from build123d import *

# Parameters (mm, degrees)
SKETCH_1_R             = 1.6
EXTRUDE_2_DEPTH        = 3
SKETCH_2_W             = 5
SKETCH_2_H             = 5.5
CUT_EXTRUDE_1_DEPTH    = 5
PATTERN_LINEAR_1_COUNT = 2
PATTERN_LINEAR_1_PITCH = 62.5


with BuildPart() as part:
    # 草图1 → 凸台-拉伸2 (new body)
    with BuildSketch(Plane.XY):
        Polygon((137.75, -25.25), (38.57, -25.25), (-17.446603057, -105.25), (137.75, -105.25), align=None)
        with Locations((36.773595123, -45.25)):
            Circle(SKETCH_1_R, mode=Mode.SUBTRACT)
        with Locations((1.763218213, -95.25)):
            Circle(SKETCH_1_R, mode=Mode.SUBTRACT)
        with Locations((127.75, -35.25)):
            Circle(SKETCH_1_R, mode=Mode.SUBTRACT)
        with Locations((127.75, -95.25)):
            Circle(SKETCH_1_R, mode=Mode.SUBTRACT)
    extrude(amount=EXTRUDE_2_DEPTH)

    # 草图2 → 切除-拉伸1 (cut)
    with BuildSketch(Plane.XY.offset(3)):
        with Locations((98.25, -97.500011017)):
            Rectangle(SKETCH_2_W, SKETCH_2_H)
        with Locations((48.25, -97.500011017)):
            Rectangle(SKETCH_2_W, SKETCH_2_H)
    cut_extrude_1 = extrude(amount=-CUT_EXTRUDE_1_DEPTH, mode=Mode.SUBTRACT)

    # 阵列(线性)1: 切除-拉伸1 ×2
    with Locations(*[(0, i * PATTERN_LINEAR_1_PITCH, 0) for i in range(1, PATTERN_LINEAR_1_COUNT)]):
        add(cut_extrude_1, mode=Mode.SUBTRACT)


solid = part.part
Input: part model. Units: mm. Frame: model coordinates. A direction names the side the tool comes from. Round coordinates to 2 decimals unless told otherwise and drop trailing zeros. Order: outer loops, then holes, each group sorted by start corner. A loop starts at its lowest first (then second) coordinate and runs counter-clockwise, first axis right, second up. Notation, with made-up numbers: (23, 7) - (31, 7) arc R19 ccw to (31, 16) - close; hole circle Ø8 at (-19.75, 36). An arc over 180 degrees is marked (long way). Answer as a JSON object with one key per item and string values. Group by question number.
(1) Cut plane C-C (y = -35.25). Return loops of the section in (x, z), then the cut area to 3 significant figures.
(2) Cut plane D-D (x = 48.5). Return loops of the section in (y, z), then the cut area to 3 significant figures.
(3) Reachability of faces 1 (the face through (100.75, -98, 2)), 2 (the face through (76, -65, 3)) from +Z, -Z, +X, -X, +Y, -Y: full face, straight path, thin tool, end or side. Return the list, or none.
(4) Material intervals for probe 1 along Y at (x, z) = (127.75, 0.65); probe 2 along X at (y, z) = (-94, 0.3); probe 3 along X at (y, z) = (-95.25, 0.75), sorted ascending. Write a range as from..to.
(5) Draft query along Y for faces 3 (the face through (89, -25.25, 1)), 4 (the face through (38.252, -45.863, 1.479)), 5 (the face through (76, -65, 0)). Return one class per face: released by +Y, released by -Y, zero draft, split by the parting line, or undercut.
(6) Cut plane A-A (x = 127.75). Return loops of the section in (y, z), then the cut area to 3 significant figures.
(7) Pin query (flat end, axial travel): P1, Ø1.5, axis at y = -57.5, z = 1.5, coming from the -X side; P2, Ø3, axis at x = 1.76, y = -95.25, coming from the +Z side; P3, Ø0.9, axis at y = -97, z = 2, coming from the -X side (3 decimals); P4, Ø0.9, axis at y = -98, z = 1, coming from the -X side. Return the tip coordinate at first contact, or that it passes through.
(8) Cut plane B-B (z = 1.3). Count the separate pieces of the cut face and the enclosed holes in it, then the cut area to 3 significant figures.
Here are the results:
{
 "1": {"outline": "(31.57, 0) - (45.75, 0) - (45.75, 3) - (31.57, 3) - close; (50.75, 0) - (95.75, 0) - (95.75, 3) - (50.75, 3) - close; (100.75, 0) - (126.15, 0) - (126.15, 3) - (100.75, 3) - close; (129.35, 0) - (137.75, 0) - (137.75, 3) - (129.35, 3) - close", "area": "279 mm^2"},
 "2": {"outline": "(-105.25, 0) - (-100.25, 0) - (-100.25, 3) - (-105.25, 3) - close; (-94.75, 0) - (-37.75, 0) - (-37.75, 3) - (-94.75, 3) - close; (-32.25, 0) - (-25.25, 0) - (-25.25, 3) - (-32.25, 3) - close", "area": "207 mm^2"},
 "3": {"face 1": "+Z, -Z", "face 2": "+Z, +X, -X, +Y, -Y"},
 "4": {"probe 1": "y = -105.25..-96.85, -93.65..-36.85, -33.65..-25.25", "probe 2": "x = -9.57..0.76, 2.76..126.75, 128.75..137.75", "probe 3": "x = -10.44..0.16, 3.36..45.75, 50.75..95.75, 100.75..126.15, 129.35..137.75"},
 "5": {"face 3": "released by +Y", "face 4": "undercut", "face 5": "zero draft"},
 "6": {"outline": "(-105.25, 0) - (-96.85, 0) - (-96.85, 3) - (-105.25, 3) - close; (-93.65, 0) - (-36.85, 0) - (-36.85, 3) - (-93.65, 3) - close; (-33.65, 0) - (-25.25, 0) - (-25.25, 3) - (-33.65, 3) - close", "area": "221 mm^2"},
 "7": {"P1": "stops at x = 15.46", "P2": "passes through", "P3": "stops at x = -11.985", "P4": "stops at x = -12.69"},
 "8": {"separate pieces": "1", "enclosed holes": "8", "area": "10,000 mm^2"}
}
